from build123d import *

# Parameters (mm, degrees)
BOSS_EXTRUDE1_DEPTH = 78.74
SHELL3_T            = -2.54
SKETCH1_3_W         = 59.69
SKETCH1_3_H         = 49.53
BOSS_EXTRUDE2_DEPTH = 2.54
BOSS_EXTRUDE3_DEPTH = 19.05
SKETCH3_W           = 45.085
SKETCH3_H           = 20.32
CUT_EXTRUDE1_DEPTH  = 3.54
SKETCH4_W           = 14.605
SKETCH4_H           = 14.605
CUT_EXTRUDE2_DEPTH  = 22.59


with BuildPart() as part:
    # Sketch1 → Boss-Extrude1 (new body)
    with BuildSketch(Plane(origin=(0, 0, 0), x_dir=(1, 0, 0), z_dir=(0, 1, 0))):
        Polygon((-50.8, 24.765), (-50.8, -24.765), (-50.8, -31.75), (50.8, -31.75), (50.8, 31.75), (-50.8, 31.75), align=None)
    extrude(amount=BOSS_EXTRUDE1_DEPTH)

    # Shell3
    shell3_openings = [part.faces().sort_by_distance(p)[0] for p in [
        (0, 78.74, 0),
    ]]
    offset(amount=SHELL3_T, openings=shell3_openings, kind=Kind.INTERSECTION)

    # Sketch1_3 → Boss-Extrude2 (add)
    with BuildSketch(Plane(origin=(0, 0, 0), x_dir=(1, 0, 0), z_dir=(0, 1, 0))):
        with Locations((-80.645, 0)):
            Rectangle(SKETCH1_3_W, SKETCH1_3_H)
    extrude(amount=BOSS_EXTRUDE2_DEPTH)

    # Sketch2 → Boss-Extrude3 (add)
    with BuildSketch(Plane(origin=(0, 2.54, 0), x_dir=(1, 0, 0), z_dir=(0, 1, 0))):
        Polygon((-50.8, 15.875), (-50.8, 18.415), (-104.14, 18.415), (-104.14, -18.415), (-50.8, -18.415), (-50.8, -15.875), (-101.6, -15.875), (-101.6, 15.875), align=None)
    extrude(amount=BOSS_EXTRUDE3_DEPTH)

    # Sketch3 → Cut-Extrude1 (cut, through all)
    with BuildSketch(Plane(origin=(0, 2.54, 0), x_dir=(1, 0, 0), z_dir=(0, 1, 0))):
        with Locations((-73.3425, 0)):
            Rectangle(SKETCH3_W, SKETCH3_H)
    extrude(amount=-CUT_EXTRUDE1_DEPTH, mode=Mode.SUBTRACT)

    # Sketch4 → Cut-Extrude2 (cut, through all)
    with BuildSketch(Plane(origin=(0, 21.59, 0), x_dir=(1, 0, 0), z_dir=(0, 1, 0))):
        with Locations((-80.645, -17.4625)):
            Rectangle(SKETCH4_W, SKETCH4_H)
    extrude(amount=-CUT_EXTRUDE2_DEPTH, mode=Mode.SUBTRACT)


solid = part.part
Could you check a few things on this model? Use its own coordinates, in mm. A direction names the side the tool comes from. Give positions to 0.01 mm unless a question says otherwise; leave off trailing zeros. Order: outer loops, then holes, each group sorted by start corner. A loop starts at its lowest first (then second) coordinate and runs counter-clockwise, first axis right, second up.
1. Thinking about a two-plate mould opening in X: for faces 5 (the flat face through (-1, 40, 29.21)), 6 (the flat face through (1, 39, -31.75)), which applies, +X half, -X half, draft (parallel to the pull), parting line (faces both ways), or undercut?
Answers below:
face 5: undercut
face 6: draft
2. Which directions (+Z, -Z, +X, -X, +Y, -Y) give clear straight access to the entire face, cutting with the end or side of a thin tool? Please do faces 1 (the flat face through (-84, 2.54, -11)), 2 (the flat face through (-87.5, 21.59, -16.5)), 3 (the flat face through (-77, 12, -18.415)), 4 (the flat face through (-62, 12, 18.415)).
Answers below:
face 1: +Y
face 2: +Z, -Z, -X, +Y
face 3: -Z, -X, +Y
face 4: +Z, -X, +Y
3. Suppose I cut it at B-B (z = 14). Write out the boundary of the cut face in (x, y).
Answers below:
outline: (-110.49, 0) - (-87.95, 0) - (-87.95, 2.54) - (-101.6, 2.54) - (-101.6, 21.59) - (-104.14, 21.59) - (-104.14, 2.54) - (-110.49, 2.54) - close; (-73.34, 0) - (50.8, 0) - (50.8, 78.74) - (48.26, 78.74) - (48.26, 2.54) - (-48.26, 2.54) - (-48.26, 78.74) - (-50.8, 78.74) - (-50.8, 2.54) - (-73.34, 2.54) - close
4. For pin 1 (4 mm diameter, centred on x = -1.5, z = 8.5, fed in from -Y); pin 2 (1.3 mm diameter, centred on x = -67.5, y = 0.5, fed in from -Z) (3 decimals); pin 3 (9.5 mm diameter, centred on x = -63.5, y = 10.5, fed in from -Z) (3 decimals); pin 4 (6 mm diameter, centred on x = -82.5, y = 11.5, fed in from +Z) (3 decimals), each with a flat end and sliding along its axis, tell me the tip position at first contact or that it passes through.
Answers below:
pin 1: stops at y = 0
pin 2: stops at z = -24.765
pin 3: stops at z = -18.415
pin 4: stops at z = -15.875
5. I need wall thicknesses on L1, parallel to X at y = 71, z = -24.5; L2, parallel to Z at x = -34.5, y = 30; L3, parallel to X at y = 6, z = 13.5. Which ranges of each line are inside material? Lowest first, please.
Answers below:
L1: x = -50.8 to -48.26, 48.26 to 50.8
L2: z = -31.75 to -29.21, 29.21 to 31.75
L3: x = -104.14 to -101.6, -50.8 to -48.26, 48.26 to 50.8
6. Suppose I cut it at D-D (z = 1). Write out the boundary of the cut face in (x, y) (3 decimals), plus the area to 3 significant figures.
Answers below:
outline: (-110.49, 0) - (-95.885, 0) - (-95.885, 2.54) - (-101.6, 2.54) - (-101.6, 21.59) - (-104.14, 21.59) - (-104.14, 2.54) - (-110.49, 2.54) - close; (-50.8, 0) - (50.8, 0) - (50.8, 78.74) - (48.26, 78.74) - (48.26, 2.54) - (-48.26, 2.54) - (-48.26, 78.74) - (-50.8, 78.74) - close
area: 731 mm2
7. Suppose I cut it at A-A (x = -54). Write out the boundary of the cut face in (y, z) (3 decimals).
Answers below:
outline: (0, -24.765) - (2.54, -24.765) - (2.54, -18.415) - (21.59, -18.415) - (21.59, -15.875) - (2.54, -15.875) - (2.54, -10.16) - (0, -10.16) - close; (0, 10.16) - (2.54, 10.16) - (2.54, 15.875) - (21.59, 15.875) - (21.59, 18.415) - (2.54, 18.415) - (2.54, 24.765) - (0, 24.765) - close
